from build123d import *

# Parameters (mm, degrees)
MAIN_PROFILE_SKETCH_R = 1.7
MAIN_EXTRUSION_DEPTH  = 2


with BuildPart() as part:
    # Main Profile Sketch → Main Extrusion (new body)
    with BuildSketch(Plane.XY.offset(50.5)):
        with BuildLine():
            Line((178, 8.195656276), (178, -8.195656276))
            ThreePointArc((178, -8.195656276), (178.9, -10.5), (178, -12.804343724))
            Line((178, -12.804343724), (178, -21))
            Line((178, -21), (222, -21))
            Line((222, -21), (222, 20))
            Line((222, 20), (178, 20))
            Line((178, 20), (178, 12.804343724))
            ThreePointArc((178, 12.804343724), (178.9, 10.5), (178, 8.195656276))
        make_face()
        with Locations((182, 0)):
            Circle(MAIN_PROFILE_SKETCH_R, mode=Mode.SUBTRACT)
        with Locations((218, 0)):
            Circle(MAIN_PROFILE_SKETCH_R, mode=Mode.SUBTRACT)
    extrude(amount=-MAIN_EXTRUSION_DEPTH)


solid = part.part
Verification items for the finished model (mm, model axes). Give positions to 0.01 mm unless a question says otherwise; leave off trailing zeros. Write each loop counter-clockwise with the first axis right and the second up, starting at its lowest first coordinate (ties: lowest second). Pieces come first, ordered by that corner, then holes. Notation, with made-up numbers: (60.5, -24.5) -> (83.5, -24.5) arc R21 ccw to (83.5, -15.5) -> close; hole circle Ø5 at (26.5, 0.5). An arc over 180 degrees is marked (long way). Use CSV: the item, a comma, the result in double quotes.
(1) Material ranges on L1, parallel to Y at x = 218, z = 49.1; L2, parallel to Y at x = 218.5, z = 48.7; L3, parallel to X at y = -11, z = 49.3, recorded low to high.
Derived:
L1,"y = -21 to -1.7, 1.7 to 20"
L2,"y = -21 to -1.62, 1.62 to 20"
L3,"x = 178.86 to 222"
(2) Sectioned sample at A-A (x = 182). Record the cut outline in (y, z), plus the area to 3 significant figures.
Derived:
outline,"(-21, 48.5) -> (-1.7, 48.5) -> (-1.7, 50.5) -> (-21, 50.5) -> close; (1.7, 48.5) -> (20, 48.5) -> (20, 50.5) -> (1.7, 50.5) -> close"
area,"75.2 mm^2"
(3) Release check for a two-part mould opening along Y. For faces 1 (the flat face through (178, -17, 50)), 2 (the flat face through (200, 20, 50)), 3 (the flat face through (200, -21, 50)), 4 (the cylindrical face through (219.62, 0.51, 49.51)) record: +Y half, -Y half, draft (parallel to the pull), parting line (faces both ways), or undercut.
Derived:
face 1,"draft"
face 2,"+Y half"
face 3,"-Y half"
face 4,"undercut"
